Part model, mm, in its own coordinate system. A direction names the side the tool comes from. Round coordinates to 2 decimals unless told otherwise and drop trailing zeros. Write each loop counter-clockwise with the first axis right and the second up, starting at its lowest first coordinate (ties: lowest second). Pieces come first, ordered by that corner, then holes.
```python
from build123d import *

# Parameters (mm, degrees)
CYLINDER041_R          = 0.7
CYLINDER041_DEPTH      = 10
CYLINDER041_ROLL_ANGLE = 90
BOX074_W               = 14
BOX074_H               = 2
BOX074_DEPTH           = 14
BOX073_W               = 10
BOX073_H               = 10
BOX073_DEPTH           = 10
CHAMFER008_SIZE        = 1


with BuildPart() as cylinder073:
    # Cylinder041 → Cylinder041 (new body)
    with BuildSketch(Plane.XY):
        Circle(CYLINDER041_R)
    extrude(amount=CYLINDER041_DEPTH)


with BuildPart() as cylinder073_1:
    # Cylinder041 roll: moved
    add(cylinder073.part.rotate(Axis((0, 0, 0), (1, 0, 0)), CYLINDER041_ROLL_ANGLE))


with BuildPart() as cylinder073_2:
    # Cylinder041 placement: moved
    add(cylinder073_1.part.moved(Location((50, 72, 53))))


with BuildPart() as cube073:
    # Box074 → Box074 (new body)
    with BuildSketch(Plane(origin=(-37, 0, 0), x_dir=(1, 0, 0), z_dir=(0, 0, 1))):
        with Locations((7, 1)):
            Rectangle(BOX074_W, BOX074_H)
    extrude(amount=BOX074_DEPTH)


with BuildPart() as cut086:
    # Box073 → Box073 (new body)
    with BuildSketch(Plane(origin=(-35, 0, 2), x_dir=(1, 0, 0), z_dir=(0, 0, 1))):
        with Locations((5, 5)):
            Rectangle(BOX073_W, BOX073_H)
    extrude(amount=BOX073_DEPTH)

    # Fusion023: union Cube073
    add(cube073.part)


with BuildPart() as cut086_1:
    # Fusion023 placement: moved
    add(cut086.part.moved(Location((80, 64, 46))))

    # Chamfer008
    chamfer008_edges = [cut086_1.edges().sort_by_distance(p)[0] for p in [
        (45, 74, 53),
        (50, 74, 48),
        (55, 74, 53),
        (50, 74, 58),
    ]]
    chamfer(chamfer008_edges, length=CHAMFER008_SIZE)

    # Cut086: cut Cylinder073
    add(cylinder073_2.part, mode=Mode.SUBTRACT)


solid = cut086_1.part
```
Q1. Cut at C-C on z = 53. Write the cut outline in (x, y), plus the area to 3 significant figures.
Values follow:
outline: (43, 64) - (49.3, 64) - (49.3, 72) - (50.7, 72) - (50.7, 64) - (57, 64) - (57, 66) - (55, 66) - (55, 73) - (54, 74) - (46, 74) - (45, 73) - (45, 66) - (43, 66) - close
area: 95.8 mm2
Q2. Cut at A-A on x = 52. Write the cut outline in (y, z), plus the area to 3 significant figures.
Values follow:
outline: (64, 46) - (66, 46) - (66, 48) - (73, 48) - (74, 49) - (74, 57) - (73, 58) - (66, 58) - (66, 60) - (64, 60) - close
area: 107 mm2
Q3. Which spindle directions (+Z, -Z, +X, -X, +Y, -Y) get a long thin tool onto all of the face, cutting with end or side? Do faces 1 (the flat face through (50, 72, 53)), 2 (the flat face through (44, 66, 53)), 3 (the flat face through (55, 69, 53)), 4 (the flat face through (50, 70, 58)), 5 (the flat face through (50, 70, 48)). Say none if no direction does.
Values follow:
face 1: -Y
face 2: +Y
face 3: +Z, -Z, +X, +Y
face 4: +Z, +X, -X, +Y
face 5: -Z, +X, -X, +Y
Q4. Mould opens along X. For faces 6 (the flat face through (45, 69, 53)), 7 (the flat face through (48, 64, 53)), 8 (the cylindrical face through (49.3, 68.1, 53)) say: +X half, -X half, draft (parallel to the pull), parting line (faces both ways), or undercut.
Values follow:
face 6: -X half
face 7: draft
face 8: undercut
Q5. Drop flat-ended pins along their axis: pin 1 (5.5 mm diameter, centred on y = 68, z = 53, fed in from -X); pin 2 (3.5 mm diameter, centred on y = 71, z = 55, fed in from +X); pin 3 (2 mm diameter, centred on y = 69, z = 55, fed in from -X); pin 4 (1.5 mm diameter, centred on x = 47.5, y = 69, fed in from +Z). Give the stop position or say it passes through.
Values follow:
pin 1: stops at x = 43
pin 2: stops at x = 55
pin 3: stops at x = 45
pin 4: stops at z = 58
Q6. Cut at B-B on y = 69. Write the cut outline in (x, z), plus the area to 3 significant figures.
Values follow:
outline: (45, 48) - (55, 48) - (55, 58) - (45, 58) - close; hole circle Ø1.4 at (50, 53)
area: 98.5 mm2
Q7. Cut at D-D on x = 50. Write the cut outline in (y, z), plus the area to 3 significant figures.
Values follow:
outline: (64, 46) - (66, 46) - (66, 48) - (73, 48) - (74, 49) - (74, 57) - (73, 58) - (66, 58) - (66, 60) - (64, 60) - (64, 53.7) - (72, 53.7) - (72, 52.3) - (64, 52.3) - close
area: 95.8 mm2
Q8. Wall check: L1, parallel to Z at x = 50, y = 70; L2, parallel to X at y = 67.5, z = 53; L3, parallel to Y at x = 56.25, z = 47.25. Give the ranges that are in metal, low to high.
Values follow:
L1: z = 48 to 52.3, 53.7 to 58
L2: x = 45 to 49.3, 50.7 to 55
L3: y = 64 to 66
